Read the model definition and answer for the solid it produces. Units are mm, in the model's axes. Round coordinates to 2 decimals unless told otherwise and drop trailing zeros. Loops run counter-clockwise (first coordinate to the right, second up) from the corner with the lowest first, then second, coordinate; pieces in that order, holes last. Notation, with made-up numbers: (-2.5, -34.75) -> (38.5, -34.75) arc R25 cw to (38.5, -11.75) -> close; hole circle Ø4 at (-0.5, 82). An arc over 180 degrees is marked (long way). Put each result on its own line as item: value.
from build123d import *

# Parameters (mm, degrees)
SKETCH_1_W          = 70
SKETCH_1_H          = 135
EXTRUDE_1_DEPTH     = 3
SKETCH_2_R          = 2.25
SKETCH_2_R_2        = 2
CUT_EXTRUDE_1_DEPTH = 153.098652197
FILLET_1_R          = 10
SKETCH_3_R          = 1.5
SKETCH_3_R_2        = 2.25
CUT_EXTRUDE_2_DEPTH = 153.098652197


with BuildPart() as part:
    # 草图1 → 凸台-拉伸1 (new body)
    with BuildSketch(Plane(origin=(0, 0, 0), x_dir=(1, 0, 0), z_dir=(0, 1, 0))):
        with Locations((35, -67.5)):
            Rectangle(SKETCH_1_W, SKETCH_1_H)
    extrude(amount=EXTRUDE_1_DEPTH)

    # 草图2 → 切除-拉伸1 (cut, through all)
    with BuildSketch(Plane(origin=(0, 3, 0), x_dir=(1, 0, 0), z_dir=(0, 1, 0))):
        with Locations(Location((15, -15, 0), (0, 0, 270))):
            Circle(SKETCH_2_R)
        with Locations(Location((55, -15, 0), (0, 0, 270))):
            Circle(SKETCH_2_R)
        with Locations(Location((15, -120, 0), (0, 0, 270))):
            Circle(SKETCH_2_R)
        with Locations(Location((55, -120, 0), (0, 0, 270))):
            Circle(SKETCH_2_R)
        with Locations(Location((35, -120, 0), (0, 0, 270))):
            Circle(SKETCH_2_R_2)
        with Locations(Location((35, -15, 0), (0, 0, 270))):
            Circle(SKETCH_2_R_2)
    extrude(amount=-CUT_EXTRUDE_1_DEPTH, mode=Mode.SUBTRACT)

    # 圆角1
    fillet_1_edges = [part.edges().sort_by_distance(p)[0] for p in [
        (0, 1.5, 0),
        (70, 1.5, 0),
        (70, 1.5, 135),
        (0, 1.5, 135),
    ]]
    fillet(fillet_1_edges, radius=FILLET_1_R)

    # 草图3 → 切除-拉伸2 (cut, through all)
    with BuildSketch(Plane.XZ):
        with Locations(Location((35, 47.5, 0), (0, 0, 270))):
            Circle(SKETCH_3_R)
        with Locations(Location((43, 31.375484503, 0), (0, 0, 270))):
            Circle(SKETCH_3_R)
        with Locations(Location((27, 31.375484503, 0), (0, 0, 270))):
            Circle(SKETCH_3_R)
        with Locations(Location((35, 66.5, 0), (0, 0, 270))):
            Circle(SKETCH_3_R_2)
    extrude(amount=-CUT_EXTRUDE_2_DEPTH, mode=Mode.SUBTRACT)


solid = part.part
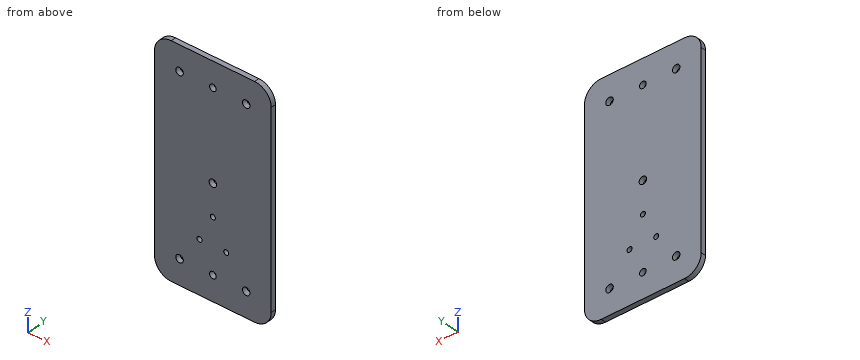
Item 1: The part is cut by section A-A (x = 35). Determine the outline of the cut face in (y, z), then the cut area to 4 significant figures.
Derived:
outline: (0, 0) -> (3, 0) -> (3, 13) -> (0, 13) -> close; (0, 17) -> (3, 17) -> (3, 46) -> (0, 46) -> close; (0, 49) -> (3, 49) -> (3, 64.25) -> (0, 64.25) -> close; (0, 68.75) -> (3, 68.75) -> (3, 118) -> (0, 118) -> close; (0, 122) -> (3, 122) -> (3, 135) -> (0, 135) -> close
area: 358.5 mm^2
Item 2: The part is cut by section B-B (z = 47.5). Determine the outline of the cut face in (x, y).
Derived:
outline: (0, 0) -> (33.5, 0) -> (33.5, 3) -> (0, 3) -> close; (36.5, 0) -> (70, 0) -> (70, 3) -> (36.5, 3) -> close
Item 3: The part is cut by section D-D (z = 120). Determine the outline of the cut face in (x, y).
Derived:
outline: (0, 0) -> (12.75, 0) -> (12.75, 3) -> (0, 3) -> close; (17.25, 0) -> (33, 0) -> (33, 3) -> (17.25, 3) -> close; (37, 0) -> (52.75, 0) -> (52.75, 3) -> (37, 3) -> close; (57.25, 0) -> (70, 0) -> (70, 3) -> (57.25, 3) -> close
Item 4: A flat-ended cylindrical pin translates along its axis: pin 1 Ø4 at (x, z) = (55, 15) entering from -Y. Find the tip coordinate at first contact, or state that the pin passes through.
Derived:
pin 1: passes through
Item 5: Find the intervals of material crossed by line 1 along Z through (x, y) = (54, 0.4); line 2 along X through (y, z) = (1.85, 120); line 3 along Z through (x, y) = (6, 0.2), in increasing order.
Derived:
line 1: z = 0 to 12.98, 17.02 to 117.98, 122.02 to 135
line 2: x = 0 to 12.75, 17.25 to 33, 37 to 52.75, 57.25 to 70
line 3: z = 0.83 to 134.17
Item 6: The part is cut by section C-C (x = 55). Determine the outline of the cut face in (y, z).
Derived:
outline: (0, 0) -> (3, 0) -> (3, 12.75) -> (0, 12.75) -> close; (0, 17.25) -> (3, 17.25) -> (3, 117.75) -> (0, 117.75) -> close; (0, 122.25) -> (3, 122.25) -> (3, 135) -> (0, 135) -> close
